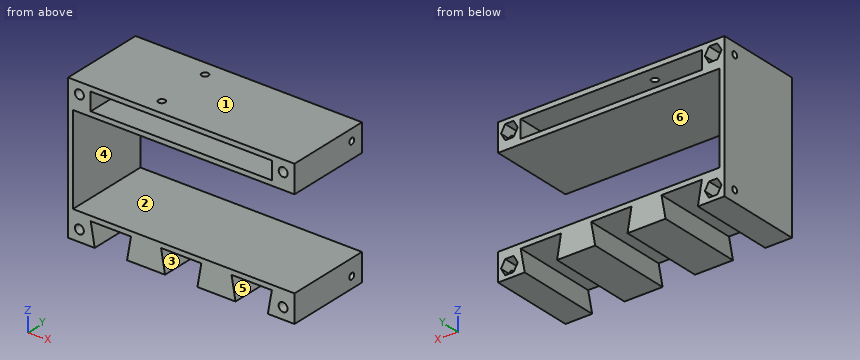
from build123d import *

# Parameters (mm, degrees)
SKETCH1_W           = 112
SKETCH1_H           = 11
BOSS_EXTRUDE2_DEPTH = 53
SKETCH2_R           = 1.9
CUT_EXTRUDE1_DEPTH  = 9.5
SKETCH3_R           = 1.9
CUT_EXTRUDE2_DEPTH  = 9.5
CUT_EXTRUDE3_REACH  = 91
SKETCH4_R           = 2.125
SKETCH5_R           = 2.75
BOSS_EXTRUDE6_DEPTH = 12


with BuildPart() as part:
    # Sketch1 → Boss-Extrude2 (new body)
    with BuildSketch(Plane(origin=(0, 0, 0), x_dir=(1, 0, 0), z_dir=(0, 1, 0))):
        Polygon((140, -17), (140, 0), (3, 0), (3, 55), (140, 55), (140, 72), (123.53142227, 72), (126, 58), (101.06284454, 58), (103.53142227, 72), (79.96857773, 72), (82.43715546, 58), (57.5, 58), (59.96857773, 72), (36.46857773, 72), (38.93715546, 58), (14, 58), (16.46857773, 72), (0, 72), (0, -17), align=None)
        with Locations((70, -8.5)):
            Rectangle(SKETCH1_W, SKETCH1_H, mode=Mode.SUBTRACT)
        Polygon((4.401923789, -5.5), (9.598076211, -5.5), (12.196152423, -10), (9.598076211, -14.5), (4.401923789, -14.5), (1.803847577, -10), align=None, mode=Mode.SUBTRACT)
        Polygon((12.196152423, 65), (9.598076211, 60.5), (4.401923789, 60.5), (1.803847577, 65), (4.401923789, 69.5), (9.598076211, 69.5), align=None, mode=Mode.SUBTRACT)
        Polygon((127.803847577, -10), (130.401923789, -5.5), (135.598076211, -5.5), (138.196152423, -10), (135.598076211, -14.5), (130.401923789, -14.5), align=None, mode=Mode.SUBTRACT)
        Polygon((135.598076211, 60.5), (130.401923789, 60.5), (127.803847577, 65), (130.401923789, 69.5), (135.598076211, 69.5), (138.196152423, 65), align=None, mode=Mode.SUBTRACT)
    extrude(amount=BOSS_EXTRUDE2_DEPTH)

    # Sketch2 → Cut-Extrude1 (cut)
    with BuildSketch(Plane(origin=(140, 0, 0), x_dir=(0, 0, -1), z_dir=(1, 0, 0))):
        with Locations((-10, 45)):
            Circle(SKETCH2_R)
        with Locations((65, 45)):
            Circle(SKETCH2_R)
    extrude(amount=-CUT_EXTRUDE1_DEPTH, mode=Mode.SUBTRACT)

    # Sketch3 → Cut-Extrude2 (cut)
    with BuildSketch(Plane.ZY):
        with Locations((-65, 45)):
            Circle(SKETCH3_R)
        with Locations((10, 45)):
            Circle(SKETCH3_R)
    extrude(amount=-CUT_EXTRUDE2_DEPTH, mode=Mode.SUBTRACT)

    # Sketch4 → Cut-Extrude3 (cut, up to next)
    with BuildSketch(Plane.XY.offset(17), mode=Mode.PRIVATE) as cut_extrude3_sk1:
        with Locations((50.5, 43.5)):
            Circle(SKETCH4_R)
    cut_extrude3_tool1 = extrude(cut_extrude3_sk1.sketch, amount=-CUT_EXTRUDE3_REACH, mode=Mode.PRIVATE) & part.part
    add(cut_extrude3_tool1.solids().sort_by_distance((50.5, 43.5, 17))[0], mode=Mode.SUBTRACT)
    # Sketch4 → Cut-Extrude3 (cut, up to next)
    with BuildSketch(Plane.XY.offset(17), mode=Mode.PRIVATE) as cut_extrude3_sk2:
        with Locations((50.5, 9.5)):
            Circle(SKETCH4_R)
    cut_extrude3_tool2 = extrude(cut_extrude3_sk2.sketch, amount=-CUT_EXTRUDE3_REACH, mode=Mode.PRIVATE) & part.part
    add(cut_extrude3_tool2.solids().sort_by_distance((50.5, 9.5, 17))[0], mode=Mode.SUBTRACT)

    # Sketch5 → Boss-Extrude6 (add)
    with BuildSketch(Plane.XZ):
        Polygon((3.904199133, -59.637915608), (10.095800867, -59.637915608), (13.191601734, -65), (10.095800867, -70.362084392), (3.904199133, -70.362084392), (0.808398266, -65), align=None)
        with Locations((7, -65)):
            Circle(SKETCH5_R, mode=Mode.SUBTRACT)
        Polygon((13.191601734, 10), (10.095800867, 15.362084392), (3.904199133, 15.362084392), (0.808398266, 10), (3.904199133, 4.637915608), (10.095800867, 4.637915608), align=None)
        with Locations((7, 10)):
            Circle(SKETCH5_R, mode=Mode.SUBTRACT)
        Polygon((139.122867425, -65.057948728), (136.03156068, -59.693272163), (129.83996112, -59.688084053), (126.739668304, -65.047572507), (129.830975049, -70.412249071), (136.022574609, -70.417437182), align=None)
        with Locations((132.931267865, -65.052760617)):
            Circle(SKETCH5_R, mode=Mode.SUBTRACT)
        Polygon((129.893819578, 4.587724599), (126.802512833, 9.952401164), (129.902805649, 15.311889618), (136.094405209, 15.306701507), (139.185711954, 9.942024942), (136.085419138, 4.582536488), align=None)
        with Locations((132.994112394, 9.947213053)):
            Circle(SKETCH5_R, mode=Mode.SUBTRACT)
    extrude(amount=-BOSS_EXTRUDE6_DEPTH)


solid = part.part
Verification items for the finished model (mm, model axes). Face numbers are marked on the shaded views. A direction names the side the tool comes from. Coordinates: 2 decimals unless noted, no trailing zeros. Write each loop counter-clockwise with the first axis right and the second up, starting at its lowest first coordinate (ties: lowest second). Pieces come first, ordered by that corner, then holes. Notation, with made-up numbers: M -1.5,81.25 L 39.5,81.25 A21 cw 39.5,107.25 Z; hole C -36.5,84 d5. An arc over 180 degrees is marked long. Use a Markdown table: item, result.
Q1. Sectioned sample at C-C, the plane y = 9.5. Count the separate pieces of the cut face and the enclosed holes in it, plus the area to 3 significant figures.
Reply:
| item | result |
|---|---|
| separate pieces | 1 |
| enclosed holes | 4 |
| area | 2,640 mm² |
Q2. Sectioned sample at D-D, the plane z = -49. Record the boundary of the cut face in (x, y).
Reply:
| item | result |
|---|---|
| outline | M 0,0 L 3,0 L 3,53 L 0,53 Z |
Q3. Draft check along X on the marked faces 4, 5 and 6. Enter one of: +X half, -X half, draft (parallel to the pull), parting line (faces both ways), or undercut.
Reply:
| item | result |
|---|---|
| face 4 | +X half |
| face 5 | undercut |
| face 6 | draft |
Q4. Go/stop test with flat-tipped pins: P1, Ø6, axis at x = 18.5, z = 3, coming from the -Y side; P2, Ø7, axis at x = 132.99, z = 9.95, coming from the +Y side. Record where each tip stops, or that it passes through.
Reply:
| item | result |
|---|---|
| P1 | stops at y = 0 |
| P2 | stops at y = 12 |
Q5. Set-up check for the marked faces 1, 2 and 3: record each of +Z, -Z, +X, -X, +Y, -Y from which the full face is reachable in a straight line by a thin tool's end or side.
Reply:
| item | result |
|---|---|
| face 1 | +Z, +X, -X, +Y, -Y |
| face 2 | +X, +Y, -Y |
| face 3 | +Y, -Y |
Q6. Sectioned sample at B-B, the plane x = 55.5. Record the boundary of the cut face in (y, z).
Reply:
| item | result |
|---|---|
| outline | M 0,-72 L 53,-72 L 53,-55 L 0,-55 Z; M 0,0 L 53,0 L 53,3 L 0,3 Z; M 0,14 L 53,14 L 53,17 L 0,17 Z |
Q7. Sectioned sample at A-A, the plane x = 7. Record the boundary of the cut face in (y, z), plus the area to 3 significant figures.
Reply:
| item | result |
|---|---|
| outline | M 0,-72 L 53,-72 L 53,-69.5 L 12,-69.5 L 12,-67.75 L 0,-67.75 Z; M 0,-62.25 L 12,-62.25 L 12,-60.5 L 53,-60.5 L 53,-55 L 0,-55 Z; M 0,0 L 53,0 L 53,5.5 L 12,5.5 L 12,7.25 L 0,7.25 Z; M 0,12.75 L 12,12.75 L 12,14.5 L 53,14.5 L 53,17 L 0,17 Z |
| area | 932 mm² |
Q8. Thickness scan on line 1 (Z direction, x = 107.5, y = 16); line 2 (Z direction, x = 134, y = 22); line 3 (Z direction, x = 1, y = 45). Record the ranges inside material, lowest first.
Reply:
| item | result |
|---|---|
| line 1 | z = -58 to -55, 0 to 3, 14 to 17 |
| line 2 | z = -72 to -69.5, -60.5 to -55, 0 to 5.5, 14.5 to 17 |
| line 3 | z = -72 to -66.9, -63.1 to 8.1, 11.9 to 17 |
